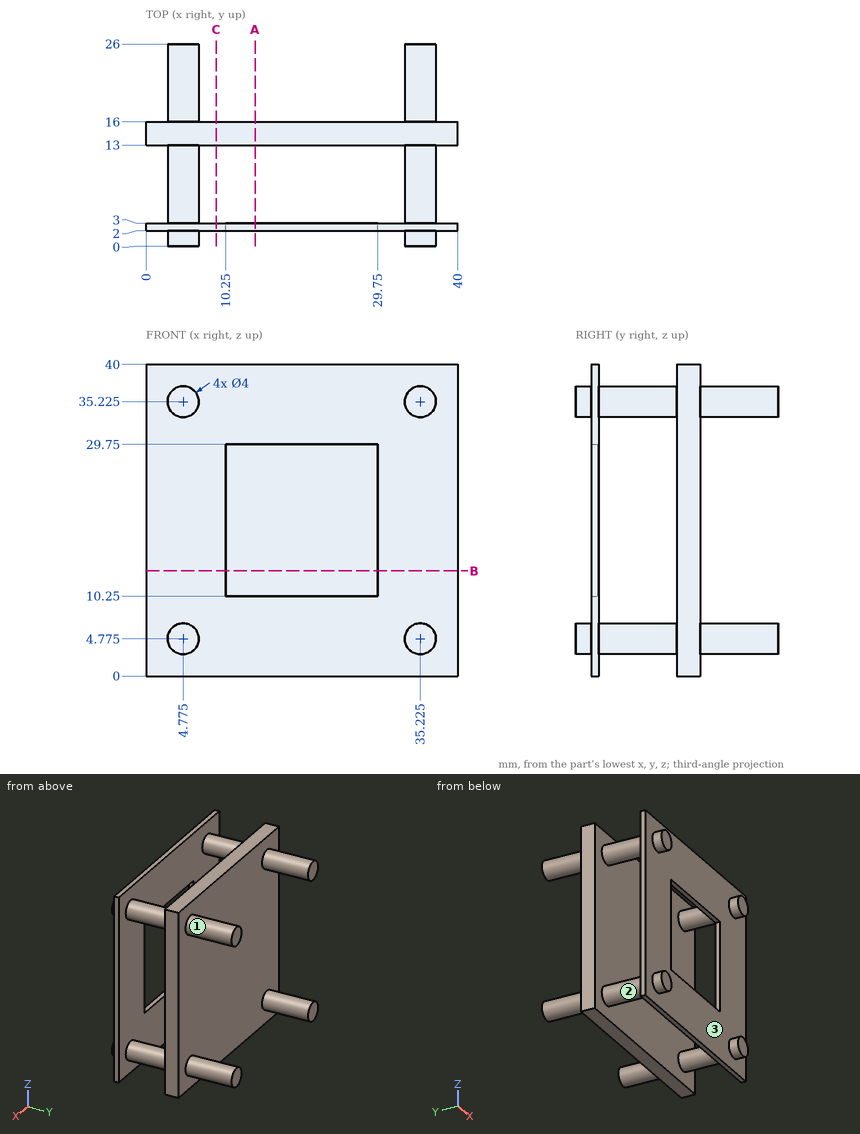
For this review, use the dimensioned drawing (mm, ordinates from the lowest corner) and the shaded views. A direction names the side the tool comes from. Give positions to 0.01 mm unless a question says otherwise; leave off trailing zeros. Order: outer loops, then holes, each group sorted by start corner. A loop starts at its lowest first (then second) coordinate and runs counter-clockwise, first axis right, second up. Notation, with made-up numbers: (10.5, 55.5) -> (14.5, 55.5) arc R19 cw to (14.5, 77.5) -> close; hole circle Ø8 at (77.5, -26). An arc over 180 degrees is marked (long way). Write item = value, one per line. Start each with the question number.
(1) Take a section at C-C (x = 9). Write out the cut boundary in (y, z).
(2) Take a section at B-B (z = 13.5). Write out the cut boundary in (x, y).
(3) For pin 1 Ø12 at (x, z) = (21, 8) entering from -Y; pin 2 Ø1.1 at (x, y) = (25, 2.5) entering from -Z; pin 3 Ø4 at (x, y) = (35.5, 18.5) entering from -Z (3 decimals); pin 4 Ø5 at (x, y) = (24, 9) entering from +Z, all flat-tipped, find the tip position at first contact; note any pin that passes through.
(4) For L1, parallel to X at y = 6, z = 35; L2, parallel to Y at x = 26, z = 33; L3, parallel to X at y = 2.5, z = 29, list the stretches that pass through material, from the lowest coordinate up. Write a range as from..to.
(5) Take a section at A-A (x = 14). Write out the cut boundary in (y, z).
(6) Tool access review of the marked faces 1, 2 and 3: name each direction out of +Z, -Z, +X, -X, +Y, -Y from which nothing blocks a thin tool from reaching the whole face with its end or side.
Returned:
q1.outline = (2, 0) -> (3, 0) -> (3, 40) -> (2, 40) -> close; (13, 0) -> (16, 0) -> (16, 40) -> (13, 40) -> close
q2.outline = (0, 2) -> (10.25, 2) -> (10.25, 3) -> (0, 3) -> close; (0, 13) -> (40, 13) -> (40, 16) -> (0, 16) -> close; (29.75, 2) -> (40, 2) -> (40, 3) -> (29.75, 3) -> close
q3.pin_1 = 2
q3.pin_2 = 0
q3.pin_3 = 2.775
q3.pin_4 = through
q4.L1 = 2.79..6.76, 33.24..37.21
q4.L2 = 2..3, 13..16
q4.L3 = 0..10.25, 29.75..40
q5.outline = (2, 0) -> (3, 0) -> (3, 10.25) -> (2, 10.25) -> close; (2, 29.75) -> (3, 29.75) -> (3, 40) -> (2, 40) -> close; (13, 0) -> (16, 0) -> (16, 40) -> (13, 40) -> close
q6.face_1 = +Y
q6.face_2 = none
q6.face_3 = -Y
